Input: part model. Units: mm. Frame: model coordinates. A direction names the side the tool comes from. Give positions to 0.01 mm unless a question says otherwise; leave off trailing zeros. Loops run counter-clockwise (first coordinate to the right, second up) from the corner with the lowest first, then second, coordinate; pieces in that order, holes last. Notation, with made-up numbers: M 15.5,-22.75 L 34.5,-22.75 A4 cw 34.5,-18.75 Z; hole C 51.5,74 d1. An arc over 180 degrees is marked long. Return JSON: item names as keys, results as strings. Group by question number.
```python
from build123d import *

# Parameters (mm, degrees)
SKETCH1_W           = 200
SKETCH1_H           = 501.6
BOSS_EXTRUDE1_DEPTH = 4
SKETCH2_W           = 200
SKETCH2_H           = 2
BOSS_EXTRUDE2_DEPTH = 47


with BuildPart() as part:
    # Sketch1 → Boss-Extrude1 (new body)
    with BuildSketch(Plane(origin=(0, 0, 0), x_dir=(0, 0, -1), z_dir=(1, 0, 0))):
        with Locations((-38.720930233, -147.020930233)):
            Rectangle(SKETCH1_W, SKETCH1_H)
    extrude(amount=BOSS_EXTRUDE1_DEPTH)

    # Sketch2 → Boss-Extrude2 (add)
    with BuildSketch(Plane.ZY):
        with Locations((38.720930233, -396.820930233)):
            Rectangle(SKETCH2_W, SKETCH2_H)
    extrude(amount=BOSS_EXTRUDE2_DEPTH)


solid = part.part
```
Item 1: Section A-A, the plane z = -11. Return loops of the section in (x, y), then the cut area to 3 significant figures.
Item 2: Section B-B, the plane x = -7.5. Return loops of the section in (y, z), then the cut area to 3 significant figures.
Item 3: Reachability of faces 1 (the face through (-23, -395.821, 37)), 2 (the face through (3, -148, 138.721)) from +Z, -Z, +X, -X, +Y, -Y: full face, straight path, thin tool, end or side. Return the list, or none.
Item 4: First-contact query: pin 1 Ø1.5 at (x, z) = (-22.5, 94.5) entering from +Y; pin 2 Ø3 at (y, z) = (-76.5, 84) entering from -X. Flat tips, straight axial feed; report the tip coordinate or a pass-through.
Item 5: Material intervals for line 1 (X direction, y = 15.5, z = 106); line 2 (Y direction, x = -13.5, z = -26.5), sorted ascending. Write a range as from..to.
Item 6: Section C-C, the plane y = 21. Return loops of the section in (x, z), then the cut area to 3 significant figures.
Answer below:
{
 "1": {"outline": "M -47,-397.82 L 4,-397.82 L 4,103.78 L 0,103.78 L 0,-395.82 L -47,-395.82 Z", "area": "2,100 mm^2"},
 "2": {"outline": "M -397.82,-61.28 L -395.82,-61.28 L -395.82,138.72 L -397.82,138.72 Z", "area": "400 mm^2"},
 "3": {"face 1": "+Z, -Z, -X, +Y", "face 2": "+Z, +X, -X, +Y, -Y"},
 "4": {"pin 1": "y = -395.82", "pin 2": "x = 0"},
 "5": {"line 1": "0..4", "line 2": "-397.82..-395.82"},
 "6": {"outline": "M 0,-61.28 L 4,-61.28 L 4,138.72 L 0,138.72 Z", "area": "800 mm^2"}
}
